Work out the finished part from the listing and answer in its coordinate system (mm). A direction names the side the tool comes from. Give positions to 0.01 mm unless a question says otherwise; leave off trailing zeros. Write each loop counter-clockwise with the first axis right and the second up, starting at its lowest first coordinate (ties: lowest second). Pieces come first, ordered by that corner, then holes.
1) Find section C-C (y = -4.5). Determine the outline of the cut face in (x, z) (3 decimals), plus the area to 3 significant figures.
2) Find section B-B (z = 0). Determine the outline of the cut face in (x, y) (3 decimals).
3) Straight lines are drawn through the part: probe 1 along X at (y, z) = (-5.75, 0) (3 decimals); probe 2 along X at (y, z) = (-17.25, -1.25). For each, find the intervals that lie inside material, in ascending order.
4) Given pin 1 Ø2 at (y, z) = (-16.5, -4.5) entering from -X; pin 2 Ø2 at (y, z) = (-15.5, 3.5) entering from +X; pin 3 Ø5 at (y, z) = (-4, -3) entering from -X, each flat-ended and moving along its own axis, determine where each tip first touches the part or whether it passes through.
5) Determine the mould class of faces 4 (the face through (-0.75, -14, 4)), 5 (the face through (-3.3, 0, 1.1)), 6 (the face through (-1.08, -10.85, -4.88)) for opening direction X: pulls with the +X half, pulls with the -X half, needs draft (parallel to the pull), parting line crosses it, or undercut.
6) Find section A-A (y = -12.75). Determine the outline of the cut face in (x, z) (3 decimals).
7) A tool of negligible diameter and unlimited length cuts with its end or side. For faces 1 (the face through (-3.255, -21.38, 0.063)), 2 (the face through (-4.1, -22, 0.4)), 3 (the face through (0.75, -14, -4)), from which of +Z, -Z, +X, -X, +Y, -Y can it reach the whole face along a straight path? Write none if from no direction.
```python
from build123d import *

# Parameters (mm, degrees)
F0_R     = 5
F0_R_2   = 3.125
F1_DEPTH = 22
F3_DEPTH = 17
F4_SIZE  = 0.2
F5_SIZE  = 0.75
F6_R     = 0.7499


# Not quite as in the source:
# - a fillet or chamfer is up to 0.001 mm smaller than in the source, because OpenCascade refuses the exact size


with BuildPart() as f1:
    # F0 (on Front) → F1 (new body)
    with BuildSketch(Plane.XZ):
        Circle(F0_R)
        Circle(F0_R_2, mode=Mode.SUBTRACT)
    extrude(amount=F1_DEPTH)

    # F2 (on face) → F3 (cut)
    with BuildSketch(Plane.XZ.offset(22)):
        with BuildLine():
            ThreePointArc((0.75, 4.9434299833), (0, 5), (-0.75, 4.9434299833))
            Line((-0.75, 4.9434299833), (-0.75, 3.0336652749))
            ThreePointArc((-0.75, 3.0336652749), (0, 3.125), (0.75, 3.0336652749))
            Line((0.75, 3.0336652749), (0.75, 4.9434299833))
        make_face()
        with BuildLine():
            ThreePointArc((-0.75, -4.9434299833), (0, -5), (0.75, -4.9434299833))
            Line((0.75, -4.9434299833), (0.75, -3.0336652749))
            ThreePointArc((0.75, -3.0336652749), (0, -3.125), (-0.75, -3.0336652749))
            Line((-0.75, -3.0336652749), (-0.75, -4.9434299833))
        make_face()
    extrude(amount=-F3_DEPTH, mode=Mode.SUBTRACT)

    # F4
    f4_edges = [f1.edges().sort_by_distance(p)[0] for p in [
        (-5, 0, 0),
        (-5, -22, 0),
        (3.791438, -22, -3.259601),
        (-3.125, 0, 0),
    ]]
    chamfer(f4_edges, length=F4_SIZE)

    # F5
    f5_edges = [f1.edges().sort_by_distance(p)[0] for p in [
        (-3.125, -22, 0),
        (2.460627, -22, -1.926379),
    ]]
    chamfer(f5_edges, length=F5_SIZE)

    # F6 (radius 0.75 in the source; OpenCascade refuses exactly that, so slightly less here)
    f6_edges = [f1.edges().sort_by_distance(p)[0] for p in [
        (0.75, -5, -3.988548),
        (-0.75, -5, 3.988548),
        (-0.75, -5, -3.988548),
        (0.75, -5, 3.988548),
    ]]
    fillet(f6_edges, radius=F6_R)


solid = f1.part
```
Results:
1. outline: circle Ø10 at (0, 0); hole circle Ø6.25 at (0, 0)
1. area: 47.9 mm2
2. outline: (-5, -21.8) - (-4.8, -22) - (-3.875, -22) - (-3.125, -21.25) - (-3.125, -0.2) - (-3.325, 0) - (-4.8, 0) - (-5, -0.2) - close; (3.125, -21.25) - (3.875, -22) - (4.8, -22) - (5, -21.8) - (5, -0.2) - (4.8, 0) - (3.325, 0) - (3.125, -0.2) - close
3. probe 1: x = -5 to -3.125, 3.125 to 5
3. probe 2: x = -4.84 to -2.86, 2.86 to 4.84
4. pin 1: stops at x = -3.57
4. pin 2: stops at x = 4.33
4. pin 3: stops at x = -4.97
5. face 4: undercut
5. face 5: needs draft
5. face 6: parting line crosses it
6. outline: (-0.75, -4.943) - (-0.75, -3.034) arc R3.125 cw to (-0.75, 3.034) - (-0.75, 4.943) arc R5 ccw to start; (0.75, -4.943) arc R5 ccw to (0.75, 4.943) - (0.75, 3.034) arc R3.125 cw to (0.75, -3.034) - close
7. face 1: -Y
7. face 2: +Z, -Z, +X, -X, -Y
7. face 3: +Z, -Z, -Y
